Input: part model. Units: mm. Frame: model coordinates. Face numbers are marked on the shaded views. A direction names the side the tool comes from. Round coordinates to 2 decimals unless told otherwise and drop trailing zeros. Loops run counter-clockwise (first coordinate to the right, second up) from the corner with the lowest first, then second, coordinate; pieces in that order, holes last.
1) Section A-A, the plane x = -4. Return loops of the section in (y, z), and give its area (3 significant figures).
2) Access query for the marked faces 3 and 4. Directions: +Z, -Z, +X, -X, +Y, -Y. A direction counts if a zero-diameter tool reaches every point of the face in a straight line with its end or side. Return the directions, or none.
3) First-contact query: pin 1 (8 mm diameter, centred on x = 5, z = -15, fed in from -Y); pin 2 (4 mm diameter, centred on x = 7.5, y = 18, fed in from -Z); pin 3 (8 mm diameter, centred on x = 6, y = -5.5, fed in from -Z). Flat tips, straight axial feed; report the tip coordinate or a pass-through.
4) Draft query along Z for the marked faces 1 and 2. Return one class per face: pulls with the +Z half, pulls with the -Z half, needs draft (parallel to the pull), parting line crosses it, or undercut.
5) Ray query, line 1 along Y through (x, z) = (-3.5, 0); line 2 along Y through (x, z) = (-0.5, 0); line 3 along Y through (x, z) = (1.25, -7.5). Return the intervals inside material, ascending.
6) Section C-C, the plane x = -7.25. Return loops of the section in (y, z), and give its area (3 significant figures).
7) Section B-B, the plane z = 8.5. State how many separate pieces and enclosed holes the cut face has, and give its area (3 significant figures).
from build123d import *

# Parameters (mm, degrees)
BASE_DEPTH          = 10
BASE_DEPTH_BACK     = 10
ESQUISSE1_R         = 25
ESQUISSE2_R         = 25
ESQUISSE2_R_2       = 23
VIDE_GORGE_DEPTH    = 7
VIDE_JANTE_DEPTH    = 20
ESQUISSE6_R         = 3
VIDE_BLOC_AXE_DEPTH = 4
CHAN_SIZE           = 2


with BuildPart() as part:
    # Esquisse1 → BASE (new, two sides: drawn at the far end of the back side and taken through both)
    with BuildSketch(Plane(origin=(0, 0, 0), x_dir=(0, 0, -1), z_dir=(1, 0, 0)).offset(-BASE_DEPTH_BACK)):
        Circle(ESQUISSE1_R)
        with BuildLine():
            Line((-1.658312395, 2.5), (1.658312395, 2.5))
            ThreePointArc((1.658312395, 2.5), (0, -3), (-1.658312395, 2.5))
        make_face(mode=Mode.SUBTRACT)
    extrude(amount=BASE_DEPTH + BASE_DEPTH_BACK)

    # Esquisse2 → VIDE GORGE (cut)
    with BuildSketch(Plane.ZY.offset(8)):
        with Locations(Location((0, 0, 0), (0, 0, 180))):
            Circle(ESQUISSE2_R)
        Circle(ESQUISSE2_R_2, mode=Mode.SUBTRACT)
    vide_gorge = extrude(amount=-VIDE_GORGE_DEPTH, mode=Mode.SUBTRACT)

    # SYM GORGE: VIDE GORGE across plane
    add(vide_gorge.mirror(Plane(origin=(0, 0, 0), x_dir=(0, 0, 1), z_dir=(1, 0, 0))), mode=Mode.SUBTRACT)

    # Esquisse4 → VIDE JANTE (cut)
    with BuildSketch(Plane(origin=(10, 0, 0), x_dir=(0, 0, -1), z_dir=(1, 0, 0))):
        with BuildLine():
            Line((-22, 0), (-5, 0))
            ThreePointArc((-5, 0), (-4.924038765, 0.868240888), (-4.698463104, 1.710100717))
            Line((-4.698463104, 1.710100717), (-20.673237657, 7.524443153))
            ThreePointArc((-20.673237657, 7.524443153), (-21.665770566, 3.820259909), (-22, 0))
        make_face()
        with BuildLine():
            ThreePointArc((-4.698463104, -1.710100717), (-4.924038765, -0.868240888), (-5, 0))
            Line((-5, 0), (-22, 0))
            ThreePointArc((-22, 0), (-21.665770566, -3.820259909), (-20.673237657, -7.524443153))
            Line((-20.673237657, -7.524443153), (-4.698463104, -1.710100717))
        make_face()
        with BuildLine():
            Line((-13.544552457, 17.336236579), (-3.078307377, 3.940053768))
            ThreePointArc((-3.078307377, 3.940053768), (-1.545084972, 4.755282581), (0.174497484, 4.996954135))
            Line((0.174497484, 4.996954135), (0.767788927, 21.986598194))
            ThreePointArc((0.767788927, 21.986598194), (-6.798373876, 20.923243358), (-13.544552457, 17.336236579))
        make_face()
        with BuildLine():
            Line((12.302243876, 18.238826596), (2.795964517, 4.145187863))
            ThreePointArc((2.795964517, 4.145187863), (4.045084972, 2.938926261), (4.80630848, 1.378186779))
            Line((4.80630848, 1.378186779), (21.147757311, 6.064021828))
            ThreePointArc((21.147757311, 6.064021828), (17.798373876, 12.93127555), (12.302243876, 18.238826596))
        make_face()
        with BuildLine():
            ThreePointArc((4.80630848, -1.378186779), (4.045084972, -2.938926261), (2.795964517, -4.145187863))
            Line((2.795964517, -4.145187863), (12.302243876, -18.238826596))
            ThreePointArc((12.302243876, -18.238826596), (17.798373876, -12.93127555), (21.147757311, -6.064021828))
            Line((21.147757311, -6.064021828), (4.80630848, -1.378186779))
        make_face()
        with BuildLine():
            ThreePointArc((0.174497484, -4.996954135), (-1.545084972, -4.755282581), (-3.078307377, -3.940053768))
            Line((-3.078307377, -3.940053768), (-13.544552457, -17.336236579))
            ThreePointArc((-13.544552457, -17.336236579), (-6.798373876, -20.923243358), (0.767788927, -21.986598194))
            Line((0.767788927, -21.986598194), (0.174497484, -4.996954135))
        make_face()
    extrude(amount=-VIDE_JANTE_DEPTH, mode=Mode.SUBTRACT)

    # Esquisse6 → VIDE BLOC AXE (cut)
    with BuildSketch(Plane.ZY.offset(10)):
        with Locations(Location((0, 0, 0), (0, 0, 180))):
            Circle(ESQUISSE6_R)
    extrude(amount=-VIDE_BLOC_AXE_DEPTH, mode=Mode.SUBTRACT)

    # CHAN
    chan_edges = [part.edges().sort_by_distance(p)[0] for p in [
        (-1, 0, -23),
        (-8, 0, -23),
        (8, 0, -23),
        (1, 0, -23),
    ]]
    chamfer(chan_edges, length=CHAN_SIZE - 0.0001)  # a hair under: the kernel refuses the full size


solid = part.part
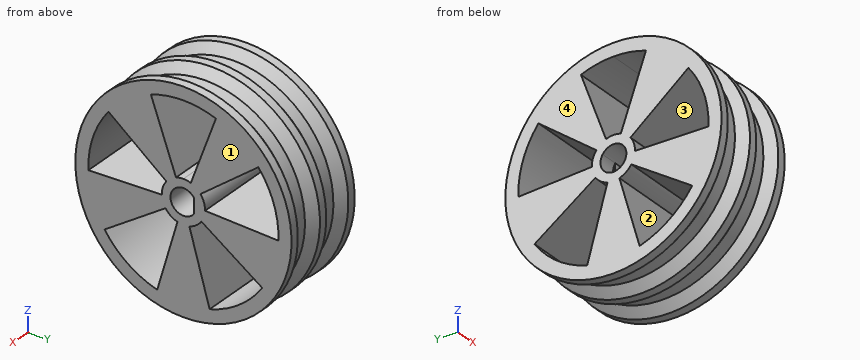
Final values:
1. outline: circle Ø46 at (0, 0); hole (-21.99, -0.77) - (-5, -0.17) arc R5 cw to (-3.94, 3.08) - (-17.34, 13.54) arc R22 ccw to start; hole (-18.24, -12.3) arc R22 ccw to (-6.06, -21.15) - (-1.38, -4.81) arc R5 cw to (-4.15, -2.8) - close; hole (-7.52, 20.67) - (-1.71, 4.7) arc R5 cw to (1.71, 4.7) - (7.52, 20.67) arc R22 ccw to start; hole (1.38, -4.81) - (6.06, -21.15) arc R22 ccw to (18.24, -12.3) - (4.15, -2.8) arc R5 cw to start; hole (2.5, -1.66) - (2.5, 1.66) arc R3 ccw (long way) to start; hole (3.94, 3.08) arc R5 cw to (5, -0.17) - (21.99, -0.77) arc R22 ccw to (17.34, 13.54) - close
1. area: 834 mm2
2. face 3: +X, -X
2. face 4: +Z, -Z, -X, +Y, -Y
3. pin 1: stops at y = -21.73
3. pin 2: stops at z = -19.16
3. pin 3: stops at z = -24.92
4. face 1: needs draft
4. face 2: undercut
5. line 1: y = -23 to -22, -5 to -3, 2.5 to 5, 22 to 23
5. line 2: y = -25 to -22, -5 to -3, 2.5 to 5, 22 to 25
5. line 3: y = -23.59 to -11.12, -2.15 to 2.15, 11.12 to 23.59
6. outline: circle Ø48.5 at (0, 0); hole (-21.99, -0.77) - (-5, -0.17) arc R5 cw to (-3.94, 3.08) - (-17.34, 13.54) arc R22 ccw to start; hole (-18.24, -12.3) arc R22 ccw to (-6.06, -21.15) - (-1.38, -4.81) arc R5 cw to (-4.15, -2.8) - close; hole (-7.52, 20.67) - (-1.71, 4.7) arc R5 cw to (1.71, 4.7) - (7.52, 20.67) arc R22 ccw to start; hole circle Ø6 at (0, 0); hole (1.38, -4.81) - (6.06, -21.15) arc R22 ccw to (18.24, -12.3) - (4.15, -2.8) arc R5 cw to start; hole (3.94, 3.08) arc R5 cw to (5, -0.17) - (21.99, -0.77) arc R22 ccw to (17.34, 13.54) - close
6. area: 1,020 mm2
7. separate pieces: 4
7. enclosed holes: 0
7. area: 397 mm2
